The model under review builds one solid part; all positions refer to its coordinate system, in mm. A direction names the side the tool comes from. Round coordinates to 2 decimals unless told otherwise and drop trailing zeros. Write each loop counter-clockwise with the first axis right and the second up, starting at its lowest first coordinate (ties: lowest second). Pieces come first, ordered by that corner, then holes. Notation, with made-up numbers: (24, -16.75) -> (59, -16.75) arc R27 ccw to (59, 18.25) -> close; hole circle Ø5 at (-19, 22). An arc over 180 degrees is marked (long way). Answer as a JSON object with one key per item and string values. Group by question number.
1) We need section B-B, the plane x = 0. Write out the cut boundary in (y, z) (3 decimals).
2) Mouldability with a two-part tool opening along X and no side actions: class faces 4 (the flat face through (93.662, 1, 11)), 5 (the cylindrical face through (54.889, 26.736, 1.377)), 6 (the flat face through (22, 1, 0)), 7 (the cylindrical face through (36.96, -23.57, 1.38)) as pulls with the +X half, pulls with the -X half, needs draft (parallel to the pull), parting line crosses it, or undercut.
3) Insertion check: pin 1 Ø4 at (x, y) = (-33.5, -15.5) entering from +Z; pin 2 Ø11 at (x, y) = (-73.5, 75.5) entering from -Z; pin 3 Ø6 at (x, y) = (-31.5, -67) entering from +Z. Each pin has a flat end and moves straight along its axis. Give the tip position at first contact, or say it passes through.
4) Machinability: for faces 1 (the cylindrical face through (-63.65, 58.37, 15.92)), 2 (the cylindrical face through (75.968, -64.875, 3.694)), 3 (the cylindrical face through (7.956, 7.296, 1.377)), which of the approach directions +Z, -Z, +X, -X, +Y, -Y give a long, thin tool a straight path to every point of the face, cutting with its end or side? Answer none if there is none.
5) We need section C-C, the plane y = -54. Count the separate pieces of the cut face and the enclosed holes in it, then the cut area to 3 significant figures.
6) To check wall thickness, follow probe 1 along X at (y, z) = (-81, 4.5); probe 2 along Y at (x, z) = (1, 12.5); probe 3 along X at (y, z) = (-73, 8). State the ranges of each line that lie inside material, in increasing order. Write a range as [from, to].
from build123d import *

# Parameters (mm, degrees)
BOSS_EXTRUDE1_DEPTH                          = 19.05
INSET_START                                  = 19.05
SKETCH4_R                                    = 86.36
INSET_RIM_DEPTH                              = 6.35
CUT_EXTRUDE1_START                           = 12.7
SKETCH9_R                                    = 69.85
CUT_EXTRUDE1_DEPTH                           = 6.35
CBORE_FOR_3_8_HEX_MACHINE_SCREW1_D           = 10.31748
CBORE_FOR_3_8_HEX_MACHINE_SCREW1_CBORE_D     = 22.225
CBORE_FOR_3_8_HEX_MACHINE_SCREW1_CBORE_DEPTH = 7.493
SKETCH12_R                                   = 10.795
CABLE_GLAND_OD_HOLES_DEPTH                   = 6.35
SKETCH13_R                                   = 69.85
CUT_EXTRUDE3_DEPTH                           = 3.556
FILLET1_R                                    = 2.54


with BuildPart() as part:
    # Sketch1 → Boss-Extrude1 (new body)
    with BuildSketch(Plane.XY):
        with BuildLine():
            Line((93.6625, 69.85), (93.6625, -69.85))
            ThreePointArc((93.6625, -69.85), (86.223012242, -87.810512242), (68.2625, -95.25))
            Line((68.2625, -95.25), (-68.2625, -95.25))
            ThreePointArc((-68.2625, -95.25), (-86.223012242, -87.810512242), (-93.6625, -69.85))
            Line((-93.6625, -69.85), (-93.6625, 69.85))
            ThreePointArc((-93.6625, 69.85), (-86.223012242, 87.810512242), (-68.2625, 95.25))
            Line((-68.2625, 95.25), (68.2625, 95.25))
            ThreePointArc((68.2625, 95.25), (86.223012242, 87.810512242), (93.6625, 69.85))
        make_face()
    extrude(amount=BOSS_EXTRUDE1_DEPTH)

    # Sketch4 → Inset Rim (cut)
    with BuildSketch(Plane.XY.offset(INSET_START)):
        Circle(SKETCH4_R)
    extrude(amount=-INSET_RIM_DEPTH, mode=Mode.SUBTRACT)

    # Sketch9 → Cut-Extrude1 (cut)
    with BuildSketch(Plane.XY.offset(CUT_EXTRUDE1_START)):
        Circle(SKETCH9_R)
    extrude(amount=-CUT_EXTRUDE1_DEPTH, mode=Mode.SUBTRACT)

    # CBORE for 3_8 Hex Machine Screw1 (through all)
    with Locations(Plane(origin=(0, 0, 0), x_dir=(-1, 0, 0), z_dir=(0, 0, -1))):
        with Locations((-74.521339476, -75.893393448), (-73.364603403, 74.715360062), (73.364603403, 74.715360062), (73.364603403, -74.715360062)):
            CounterBoreHole(CBORE_FOR_3_8_HEX_MACHINE_SCREW1_D / 2, CBORE_FOR_3_8_HEX_MACHINE_SCREW1_CBORE_D / 2, CBORE_FOR_3_8_HEX_MACHINE_SCREW1_CBORE_DEPTH)

    # Sketch12 → Cable Gland OD Holes (cut)
    with BuildSketch(Plane(origin=(0, 0, 0), x_dir=(-1, 0, 0), z_dir=(0, 0, -1))):
        Circle(SKETCH12_R)
        with Locations((19.440318364, 46.933080252)):
            Circle(SKETCH12_R)
        with Locations((46.933080827, 19.440319753)):
            Circle(SKETCH12_R)
        with Locations((46.933082215, -19.440316401)):
            Circle(SKETCH12_R)
        with Locations((19.440321716, -46.933078863)):
            Circle(SKETCH12_R)
        with Locations((-19.440314437, -46.933080252)):
            Circle(SKETCH12_R)
        with Locations((-46.9330769, -19.440319753)):
            Circle(SKETCH12_R)
        with Locations((-46.933078288, 19.440316401)):
            Circle(SKETCH12_R)
        with Locations((-19.440317789, 46.933078863)):
            Circle(SKETCH12_R)
    extrude(amount=-CABLE_GLAND_OD_HOLES_DEPTH, mode=Mode.SUBTRACT)

    # Sketch13 → Cut-Extrude3 (cut)
    with BuildSketch(Plane.XY.offset(6.35)):
        Circle(SKETCH13_R)
    extrude(amount=-CUT_EXTRUDE3_DEPTH, mode=Mode.SUBTRACT)

    # Fillet1
    fillet1_edges = [part.edges().sort_by_distance(p)[0] for p in [
        (93.6625, 0, 0),
        (86.223012242, -87.810512242, 0),
        (0, -95.25, 0),
        (-86.223012242, -87.810512242, 0),
        (-69.85, 0, 2.794),
        (-93.6625, 0, 0),
        (-86.223012242, 87.810512242, 0),
        (0, 95.25, 0),
        (86.223012242, 87.810512242, 0),
    ]]
    fillet(fillet1_edges, radius=FILLET1_R)


solid = part.part
Here are the results:
{
 "1": {"outline": "(-95.25, 2.54) arc R2.54 ccw to (-92.71, 0) -> (-10.795, 0) -> (-10.795, 2.794) -> (-67.31, 2.794) arc R2.54 cw to (-69.85, 5.334) -> (-69.85, 12.7) -> (-86.36, 12.7) -> (-86.36, 19.05) -> (-95.25, 19.05) -> close; (10.795, 0) -> (92.71, 0) arc R2.54 ccw to (95.25, 2.54) -> (95.25, 19.05) -> (86.36, 19.05) -> (86.36, 12.7) -> (69.85, 12.7) -> (69.85, 5.334) arc R2.54 cw to (67.31, 2.794) -> (10.795, 2.794) -> close"},
 "2": {"face 4": "pulls with the +X half", "face 5": "undercut", "face 6": "needs draft", "face 7": "undercut"},
 "3": {"pin 1": "stops at z = 2.79", "pin 2": "stops at z = 7.49", "pin 3": "stops at z = 12.7"},
 "4": {"face 1": "+Z", "face 2": "-Z", "face 3": "+Z, -Z"},
 "5": {"separate pieces": "3", "enclosed holes": "0", "area": "1,750 mm^2"},
 "6": {"probe 1": "x = [-91.08, -82.53], [-64.2, 64.65], [84.39, 91.08]", "probe 2": "y = [-95.25, -69.84], [69.84, 95.25]", "probe 3": "x = [-93.47, -78.23], [-68.5, 70.25], [78.79, 93.47]"}
}
